Verification items for the finished model (mm, model axes). Face numbers are marked on the shaded views. A direction names the side the tool comes from. Give positions to 0.01 mm unless a question says otherwise; leave off trailing zeros. Write each loop counter-clockwise with the first axis right and the second up, starting at its lowest first coordinate (ties: lowest second). Pieces come first, ordered by that corner, then holes. Notation, with made-up numbers: (55.5, -10.75) -> (85.5, -10.75) arc R17 cw to (85.5, 1.25) -> close; hole circle Ø6 at (14, 40.25). An arc over 180 degrees is marked (long way). Use one line per item in the form item = value. Start each with the question number.
(1) Scan lines: L1, parallel to Z at x = 26.5, y = 10.5; L2, parallel to Y at x = 26, z = 30.5 (3 decimals); L3, parallel to Z at x = 43, y = 2. Record each from-to range of solid material in increasing order.
(2) Section check C-C, the plane x = 39.5. Record the cut outline in (y, z) (3 decimals), plus the area to 3 significant figures.
(3) Release check for a two-part mould opening along Z. For the marked faces 1, 2 and 3 record: pulls with the +Z half, pulls with the -Z half, needs draft (parallel to the pull), parting line crosses it, or undercut.
(4) Depth check by flat-ended pin: pin 1 Ø2.5 at (x, z) = (25, 14.5) entering from -Y; pin 2 Ø6 at (x, y) = (42.5, 32) entering from +Z; pin 3 Ø4.5 at (x, y) = (23.5, 6.5) entering from +Z. Enter the tip coordinate at first touch or a pass-through.
(5) Section check A-A, the plane z = 43. Record the cut outline in (x, y) (3 decimals), plus the area to 3 significant figures.
(6) Section check B-B, the plane x = 25.4. Record the cut outline in (y, z) (3 decimals), plus the area to 3 significant figures.
(7) Set-up check for the marked faces 4, 5 and 6: record each of +Z, -Z, +X, -X, +Y, -Y from which the full face is reachable in a straight line by a thin tool's end or side.
(8) Section check D-D, the plane y = 18. Record the cut outline in (x, z), plus the area to 3 significant figures.
from build123d import *

# Parameters (mm, degrees)
BOSS_EXTRUDE1_DEPTH = 50.8
CUT_EXTRUDE1_DEPTH  = 80.881384721
FILLET1_R           = 5.08


with BuildPart() as part:
    # Sketch1 → Boss-Extrude1 (new body)
    with BuildSketch(Plane(origin=(0, 0, 0), x_dir=(0, 0, -1), z_dir=(1, 0, 0))):
        Polygon((0, 0), (-11.43, 0), (-11.43, 15.24), (-19.05, 15.24), (-19.05, 0), (-50.8, 0), (-50.8, 3.175), (-24.13, 3.175), (-24.13, 38.1), (0, 38.1), align=None)
    extrude(amount=BOSS_EXTRUDE1_DEPTH)

    # Sketch2 → Cut-Extrude1 (cut, through all)
    with BuildSketch(Plane(origin=(0, 3.175, 0), x_dir=(1, 0, 0), z_dir=(0, 1, 0))):
        with BuildLine():
            Line((28.1686, -34.29), (28.1686, -44.45))
            ThreePointArc((28.1686, -44.45), (25.4, -47.2186), (22.6314, -44.45))
            Line((22.6314, -44.45), (22.6314, -34.29))
            ThreePointArc((22.6314, -34.29), (25.4, -31.5214), (28.1686, -34.29))
        make_face()
    extrude(amount=-CUT_EXTRUDE1_DEPTH, mode=Mode.SUBTRACT)

    # Fillet1
    fillet1_edges = [part.edges().sort_by_distance(p)[0] for p in [
        (25.4, 3.175, 24.13),
        (25.4, 38.1, 24.13),
    ]]
    fillet(fillet1_edges, radius=FILLET1_R)


solid = part.part
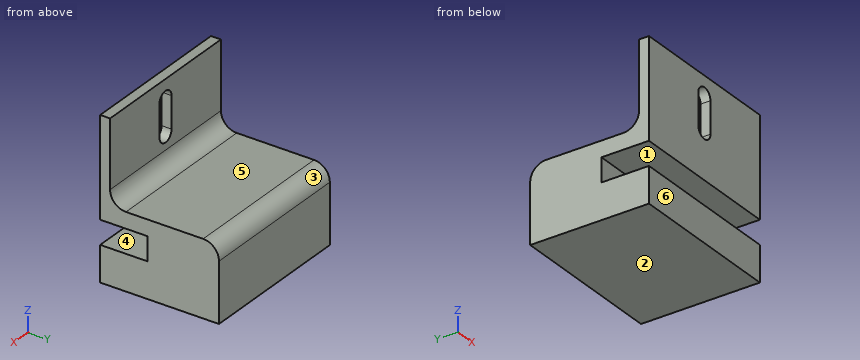
Completed:
q1.L1 = 0 to 11.43, 19.05 to 24.13
q1.L2 = 0 to 3.175
q1.L3 = 0 to 11.43, 19.05 to 50.8
q2.outline = (0, 0) -> (38.1, 0) -> (38.1, 19.05) arc R5.08 ccw to (33.02, 24.13) -> (8.255, 24.13) arc R5.08 cw to (3.175, 29.21) -> (3.175, 50.8) -> (0, 50.8) -> (0, 19.05) -> (15.24, 19.05) -> (15.24, 11.43) -> (0, 11.43) -> close
q2.area = 888 mm²
q3.face_1 = undercut
q3.face_2 = pulls with the -Z half
q3.face_3 = pulls with the +Z half
q4.pin_1 = 15.24
q4.pin_2 = 24.13
q4.pin_3 = 26.08
q5.outline = (0, 0) -> (22.631, 0) -> (22.631, 3.175) -> (0, 3.175) -> close; (28.169, 0) -> (50.8, 0) -> (50.8, 3.175) -> (28.169, 3.175) -> close
q5.area = 144 mm²
q6.outline = (0, 0) -> (38.1, 0) -> (38.1, 19.05) arc R5.08 ccw to (33.02, 24.13) -> (8.255, 24.13) arc R5.08 cw to (3.175, 29.21) -> (3.175, 31.521) -> (0, 31.521) -> (0, 19.05) -> (15.24, 19.05) -> (15.24, 11.43) -> (0, 11.43) -> close; (0, 47.219) -> (3.175, 47.219) -> (3.175, 50.8) -> (0, 50.8) -> close
q6.area = 838 mm²
q7.face_4 = +X, -X, -Y
q7.face_5 = +Z, +X, -X, +Y
q7.face_6 = +Z, -Z, +X, -X, -Y
q8.outline = (0, 0) -> (50.8, 0) -> (50.8, 24.13) -> (0, 24.13) -> close
q8.area = 1,230 mm²
